For this review, take the finished solid that the model builds, in its own axes (mm). Face numbers are marked on the shaded views. A direction names the side the tool comes from. Round coordinates to 2 decimals unless told otherwise and drop trailing zeros. Write each loop counter-clockwise with the first axis right and the second up, starting at its lowest first coordinate (ties: lowest second). Pieces come first, ordered by that corner, then holes.
Autodesk Fusion 360 part; units mm, degrees
sketch "Sketch1" plane through (0, 0, 0) normal (0, 1, 0) x (1, 0, 0)
  line L0 (0, 0) -> (10, 0)
  line L1 (10, 0) -> (10, -40)
  line L2 (10, -40) -> (0, -40)
  line L3 (0, -40) -> (0, 0)
  dimension "d1" = 10
  dimension "d2" = 40
extrude "Extrude1" add sketch "Sketch1" along normal blind 210
sketch "Sketch2" plane through (0, 210, 0) normal (0, 1, 0) x (-1, 0, 0)
  line L0 (0, 40) -> (-10, 40)
  line L1 (-10, 40) -> (-10, 0)
  line L2 (-10, 0) -> (0, 0)
  line L3 (0, 0) -> (0, 40)
  line L4 (0, 15) -> (3, 15)
  line L5 (3, 15) -> (3, 25)
  line L6 (3, 25) -> (0, 25)
  line L7 (0, 25) -> (0, 15)
  line L8 (-10, 0) -> (-13, 0)
  line L9 (-13, 0) -> (-13, 10)
  line L10 (-13, 10) -> (-10, 10)
  line L11 (-10, 10) -> (-10, 0)
  line L12 (-10, 30) -> (-13, 30)
  line L13 (-13, 30) -> (-13, 40)
  line L14 (-13, 40) -> (-10, 40)
  line L15 (-10, 40) -> (-10, 30)
  dimension "d5" = 3
  dimension "d10" = 3
  dimension "d11" = 3
extrude "Extrude2" add sketch "Sketch2" along normal blind 10 and the other way blind 10 contours L1 L12 L13 L14 L15 | L3 L4 L5 L6 L7 | L1 L8 L9 L10 L11
sketch "Sketch3" plane through (10, 0, 0) normal (1, 0, 0) x (0, 0, -1)
  line L0 (-10, 200) -> (-10, 210)
  line L1 (-10, 210) -> (-30, 210)
  line L2 (-30, 210) -> (-30, 200)
  line L3 (-30, 200) -> (-40, 200)
  line L4 (-40, 200) -> (-40, 0)
  line L5 (-40, 0) -> (0, 0)
  line L6 (0, 0) -> (0, 200)
  line L7 (0, 200) -> (-10, 200)
sketch "Sketch4" plane through (0, 0, 40) normal (0, 0, 1) x (1, 0, 0)
  line L0 (0, 0) -> (10, 0)
  line L1 (10, 0) -> (10, 200)
  line L2 (10, 200) -> (13, 200)
  line L3 (13, 200) -> (13, 220)
  line L4 (13, 220) -> (10, 220)
  line L5 (10, 220) -> (10, 210)
  line L6 (10, 210) -> (0, 210)
  line L7 (0, 210) -> (0, 0)
  line L8 (10, 15) -> (4, 15)
  line L9 (4, 15) -> (4, 20)
  line L10 (4, 20) -> (10, 20)
  line L11 (10, 20) -> (10, 15)
  line L12 (4, 20) -> (7, 20)
  line L13 (7, 20) -> (7, 22)
  line L14 (7, 22) -> (4, 22)
  line L15 (4, 22) -> (4, 20)
  line L16 (4, 22) -> (10, 22)
  line L17 (10, 22) -> (10, 24)
  line L18 (10, 24) -> (4, 24)
  line L19 (4, 24) -> (4, 22)
  line L20 (4, 44) -> (10, 44)
  line L21 (4, 46) -> (10, 46)
  line L22 (7, 44) -> (7, 46)
  line L23 (4, 46) -> (4, 44)
  line L24 (10, 48) -> (4, 48)
  line L25 (4, 39) -> (4, 44)
  line L26 (10, 39) -> (4, 39)
  line L27 (10, 44) -> (10, 39)
  line L28 (10, 46) -> (10, 48)
  line L29 (4, 48) -> (4, 46)
  line L30 (4, 68) -> (10, 68)
  line L31 (4, 70) -> (10, 70)
  line L32 (7, 68) -> (7, 70)
  line L33 (4, 70) -> (4, 68)
  line L34 (10, 72) -> (4, 72)
  line L35 (4, 63) -> (4, 68)
  line L36 (10, 63) -> (4, 63)
  line L37 (10, 68) -> (10, 63)
  line L38 (10, 70) -> (10, 72)
  line L39 (4, 72) -> (4, 70)
  line L40 (4, 92) -> (10, 92)
  line L41 (4, 94) -> (10, 94)
  line L42 (7, 92) -> (7, 94)
  line L43 (4, 94) -> (4, 92)
  line L44 (10, 96) -> (4, 96)
  line L45 (4, 87) -> (4, 92)
  line L46 (10, 87) -> (4, 87)
  line L47 (10, 92) -> (10, 87)
  line L48 (10, 94) -> (10, 96)
  line L49 (4, 96) -> (4, 94)
  line L50 (4, 116) -> (10, 116)
  line L51 (4, 118) -> (10, 118)
  line L52 (7, 116) -> (7, 118)
  line L53 (4, 118) -> (4, 116)
  line L54 (10, 120) -> (4, 120)
  line L55 (4, 111) -> (4, 116)
  line L56 (10, 111) -> (4, 111)
  line L57 (10, 116) -> (10, 111)
  line L58 (10, 118) -> (10, 120)
  line L59 (4, 120) -> (4, 118)
  line L60 (4, 140) -> (10, 140)
  line L61 (4, 142) -> (10, 142)
  line L62 (7, 140) -> (7, 142)
  line L63 (4, 142) -> (4, 140)
  line L64 (10, 144) -> (4, 144)
  line L65 (4, 135) -> (4, 140)
  line L66 (10, 135) -> (4, 135)
  line L67 (10, 140) -> (10, 135)
  line L68 (10, 142) -> (10, 144)
  line L69 (4, 144) -> (4, 142)
  line L70 (4, 164) -> (10, 164)
  line L71 (4, 166) -> (10, 166)
  line L72 (7, 164) -> (7, 166)
  line L73 (4, 166) -> (4, 164)
  line L74 (10, 168) -> (4, 168)
  line L75 (4, 159) -> (4, 164)
  line L76 (10, 159) -> (4, 159)
  line L77 (10, 164) -> (10, 159)
  line L78 (10, 166) -> (10, 168)
  line L79 (4, 168) -> (4, 166)
  line L80 (4, 188) -> (10, 188)
  line L81 (4, 190) -> (10, 190)
  line L82 (7, 188) -> (7, 190)
  line L83 (4, 190) -> (4, 188)
  line L84 (10, 192) -> (4, 192)
  line L85 (4, 183) -> (4, 188)
  line L86 (10, 183) -> (4, 183)
  line L87 (10, 188) -> (10, 183)
  line L88 (10, 190) -> (10, 192)
  line L89 (4, 192) -> (4, 190)
  dimension "d12" = 5
  dimension "d13" = 2
  dimension "d14" = 2
  dimension "d15" = 6
  dimension "d16" = 3
  dimension "d17" = 15
  dimension "d20" = 168
  dimension "d21" = 0
extrude "Extrude3" cut sketch "Sketch4" against normal blind 30 contours L1 L8 L9 L10 L11 L12 | L1 L10 L13 L16 | L1 L14 L16 L17 L18 L19 | L10 L12 L13 L14 L15 L16 | L1 L20 L25 L26 L27 | L1 L20 L21 L22 | L1 L81 L84 L88 L89 | L1 L21 L24 L28 L29 | L20 L21 L22 L23 | L1 L80 L81 L82 | L1 L80 L85 L86 L87 | L80 L81 L82 L83 | L1 L30 L35 L36 L37 | L1 L30 L31 L32 | L1 L71 L74 L78 L79 | L1 L31 L34 L38 L39 | L30 L31 L32 L33 | L1 L70 L71 L72 | L1 L70 L75 L76 L77 | L70 L71 L72 L73 | L1 L40 L45 L46 L47 | L1 L40 L41 L42 | L1 L61 L64 L68 L69 | L1 L41 L44 L48 L49 | L40 L41 L42 L43 | L1 L60 L61 L62 | L1 L60 L65 L66 L67 | L60 L61 L62 L63 | L1 L50 L55 L56 L57 | L1 L50 L51 L52 | L1 L51 L54 L58 L59 | L50 L51 L52 L53
sketch "Sketch6" plane through (0, 0, 40) normal (0, 0, 1) x (1, 0, 0)
  line L0 (4, 120) -> (10, 120)
  line L1 (10, 120) -> (10, 135)
  line L2 (10, 135) -> (4, 135)
  line L3 (4, 135) -> (4, 144)
  line L4 (4, 144) -> (10, 144)
  line L5 (10, 144) -> (10, 159)
  line L6 (10, 159) -> (4, 159)
  line L7 (4, 159) -> (4, 168)
  line L8 (4, 168) -> (10, 168)
  line L9 (10, 168) -> (10, 183)
  line L10 (10, 183) -> (4, 183)
  line L11 (4, 183) -> (4, 192)
  line L12 (4, 192) -> (10, 192)
  line L13 (10, 192) -> (10, 200)
  line L14 (10, 200) -> (13, 200)
  line L15 (13, 200) -> (13, 220)
  line L16 (13, 220) -> (10, 220)
  line L17 (10, 220) -> (10, 210)
  line L18 (10, 210) -> (0, 210)
  line L19 (0, 210) -> (0, 0)
  line L20 (0, 0) -> (10, 0)
  line L21 (10, 0) -> (10, 15)
  line L22 (10, 15) -> (4, 15)
  line L23 (4, 15) -> (4, 24)
  line L24 (4, 24) -> (10, 24)
  line L25 (10, 24) -> (10, 39)
  line L26 (10, 39) -> (4, 39)
  line L27 (4, 39) -> (4, 48)
  line L28 (4, 48) -> (10, 48)
  line L29 (10, 48) -> (10, 63)
  line L30 (10, 63) -> (4, 63)
  line L31 (4, 63) -> (4, 72)
  line L32 (4, 72) -> (10, 72)
  line L33 (10, 72) -> (10, 87)
  line L34 (10, 87) -> (4, 87)
  line L35 (4, 87) -> (4, 96)
  line L36 (4, 96) -> (10, 96)
  line L37 (10, 96) -> (10, 111)
  line L38 (10, 111) -> (4, 111)
  line L39 (4, 111) -> (4, 120)
  line L40 (4, 192) -> (6, 192)
  line L41 (6, 192) -> (6, 194)
  line L42 (6, 194) -> (4, 194)
  line L43 (4, 194) -> (4, 192)
  line L44 (4, 183) -> (6, 183)
  line L45 (6, 183) -> (6, 181)
  line L46 (6, 181) -> (4, 181)
  line L47 (4, 181) -> (4, 183)
  line L48 (6, 157) -> (4, 157)
  line L49 (6, 159) -> (6, 157)
  line L50 (4, 159) -> (6, 159)
  line L51 (4, 157) -> (4, 159)
  line L52 (4, 168) -> (6, 168)
  line L53 (6, 168) -> (6, 170)
  line L54 (6, 170) -> (4, 170)
  line L55 (4, 170) -> (4, 168)
  line L56 (6, 133) -> (4, 133)
  line L57 (6, 135) -> (6, 133)
  line L58 (4, 135) -> (6, 135)
  line L59 (4, 133) -> (4, 135)
  line L60 (4, 144) -> (6, 144)
  line L61 (6, 144) -> (6, 146)
  line L62 (6, 146) -> (4, 146)
  line L63 (4, 146) -> (4, 144)
  line L64 (6, 109) -> (4, 109)
  line L65 (6, 111) -> (6, 109)
  line L66 (4, 111) -> (6, 111)
  line L67 (4, 109) -> (4, 111)
  line L68 (4, 120) -> (6, 120)
  line L69 (6, 120) -> (6, 122)
  line L70 (6, 122) -> (4, 122)
  line L71 (4, 122) -> (4, 120)
  line L72 (6, 85) -> (4, 85)
  line L73 (6, 87) -> (6, 85)
  line L74 (4, 87) -> (6, 87)
  line L75 (4, 85) -> (4, 87)
  line L76 (4, 96) -> (6, 96)
  line L77 (6, 96) -> (6, 98)
  line L78 (6, 98) -> (4, 98)
  line L79 (4, 98) -> (4, 96)
  line L80 (6, 61) -> (4, 61)
  line L81 (6, 63) -> (6, 61)
  line L82 (4, 63) -> (6, 63)
  line L83 (4, 61) -> (4, 63)
  line L84 (4, 72) -> (6, 72)
  line L85 (6, 72) -> (6, 74)
  line L86 (6, 74) -> (4, 74)
  line L87 (4, 74) -> (4, 72)
  line L88 (6, 37) -> (4, 37)
  line L89 (6, 39) -> (6, 37)
  line L90 (4, 39) -> (6, 39)
  line L91 (4, 37) -> (4, 39)
  line L92 (4, 48) -> (6, 48)
  line L93 (6, 48) -> (6, 50)
  line L94 (6, 50) -> (4, 50)
  line L95 (4, 50) -> (4, 48)
  line L96 (6, 13) -> (4, 13)
  line L97 (6, 15) -> (6, 13)
  line L98 (4, 15) -> (6, 15)
  line L99 (4, 13) -> (4, 15)
  line L100 (4, 24) -> (6, 24)
  line L101 (6, 24) -> (6, 26)
  line L102 (6, 26) -> (4, 26)
  line L103 (4, 26) -> (4, 24)
  dimension "d31" = 2
  dimension "d32" = 2
  dimension "d33" = 2
  dimension "d34" = 2
  dimension "d37" = -168
  dimension "d38" = 0
extrude "Extrude5" cut sketch "Sketch6" against normal blind 30 contours L0 L68 L69 L70 L71 | L38 L64 L65 L66 L67 | L2 L56 L57 L58 L59 | L36 L76 L77 L78 L79 | L4 L60 L61 L62 L63 | L34 L72 L73 L74 L75 | L6 L48 L49 L50 L51 | L32 L84 L85 L86 L87 | L8 L52 L53 L54 L55 | L30 L80 L81 L82 L83 | L10 L44 L45 L46 L47 | L28 L92 L93 L94 L95 | L12 L40 L41 L42 L43 | L26 L88 L89 L90 L91 | L24 L100 L101 L102 L103 | L22 L96 L97 L98 L99
sketch "Sketch7" plane through (13, 0, 0) normal (1, 0, 0) x (0, 0, -1)
  line L0 (-30, 200) -> (-30, 220)
  line L1 (-30, 220) -> (-40, 220)
  line L2 (-40, 220) -> (-40, 200)
  line L3 (-40, 200) -> (-30, 200)
  circle A0 centre (-35, 215) radius 1.7
  circle A1 centre (-5, 215) radius 1.7
  circle A2 centre (-20, 215) radius 1.7
  line L4 (-35, 220) -> (-35, 200) construction
  line L5 (-5, 220) -> (-5, 200) construction
  line L6 (-20, 220) -> (-20, 210) construction
  line L7 (-25, 220) -> (-15, 220)
  line L8 (-10, 220) -> (0, 220)
  dimension "d41" = 3.4
  dimension "d42" = 3.4
  dimension "d43" = 3.4
  dimension "d44" = 5
  dimension "d45" = 5
  dimension "d46" = 5
extrude "Extrude6" cut sketch "Sketch7" against normal blind 40 contours A0 | A1 | A2
sketch "Sketch8" plane through (10, 0, 0) normal (1, 0, 0) x (0, 0, -1)
  circle A0 centre (-35, 5) radius 1.7
  circle A1 centre (-20, 5) radius 1.7
  circle A2 centre (-5, 5) radius 1.7
  line L0 (-40, 0) -> (0, 0)
  line L1 (-40, 200) -> (-40, 0)
  line L2 (0, 0) -> (0, 200)
  dimension "d49" = 3.4
  dimension "d50" = 3.4
  dimension "d51" = 3.4
  dimension "d52" = 5
  dimension "d53" = 5
  dimension "d54" = 5
  dimension "d55" = 5
  dimension "d56" = 5
  dimension "d57" = 20
extrude "Extrude7" cut sketch "Sketch8" against normal blind 37
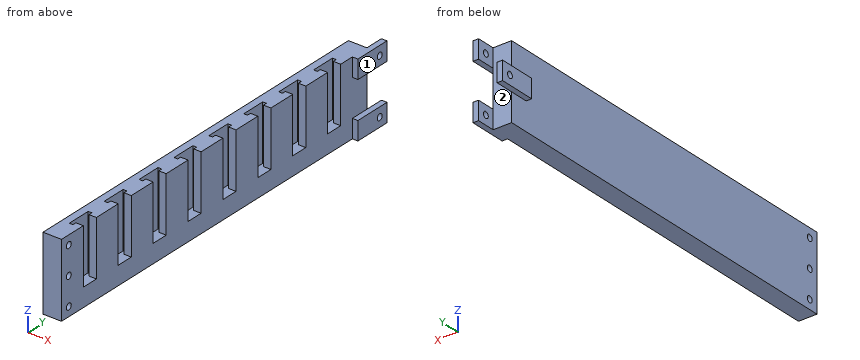
(1) We need section A-A, the plane y = 114. Give the boundary of the cut face in (x, z).
Geometry check:
outline: (0, 0) - (10, 0) - (10, 10) - (4, 10) - (4, 40) - (0, 40) - close
(2) We need section B-B, the plane y = 29. Give the boundary of the cut face in (x, z), and give its area (3 significant figures).
Geometry check:
outline: (0, 0) - (10, 0) - (10, 40) - (0, 40) - close
area: 400 mm2
(3) For pin 1 Ø3 at (x, z) = (9.5, 17.5) entering from +Y; pin 2 Ø0.6 at (y, z) = (62, 32.5) entering from -X; pin 3 Ø3 at (y, z) = (214, 36.5) entering from -X, all flat-tipped, find the tip position at first contact; note any pin that passes through.
Geometry check:
pin 1: stops at y = 210
pin 2: stops at x = 0
pin 3: stops at x = 10
(4) For line 1 along Z through (x, y) = (12.15, 215); line 2 along X through (y, z) = (182.5, 16); line 3 along Y through (x, z) = (12.25, 9), list the stretches that pass through material, from the lowest coordinate up.
Geometry check:
line 1: z = 0 to 3.3, 6.7 to 10, 30 to 33.3, 36.7 to 40
line 2: x = 0 to 4, 6 to 10
line 3: y = 200 to 220
(5) For the marked faces 1 and 2, list the 3-axis set-ups (+Z, -Z, +X, -X, +Y, -Y) from which the entire face can be reached by the end or side of a thin tool; tool diameter is ignored.
Geometry check:
face 1: +Z, -Z, +X, +Y, -Y
face 2: +Z, -Z, +Y
